Geometry: see drawing. Coordinates: mm, zero at the bounding-box minimum. A direction names the side the tool comes from. Give positions to 0.01 mm unless a question says otherwise; leave off trailing zeros. Write each loop counter-clockwise with the first axis right and the second up, starting at its lowest first coordinate (ties: lowest second). Pieces come first, ordered by that corner, then holes.
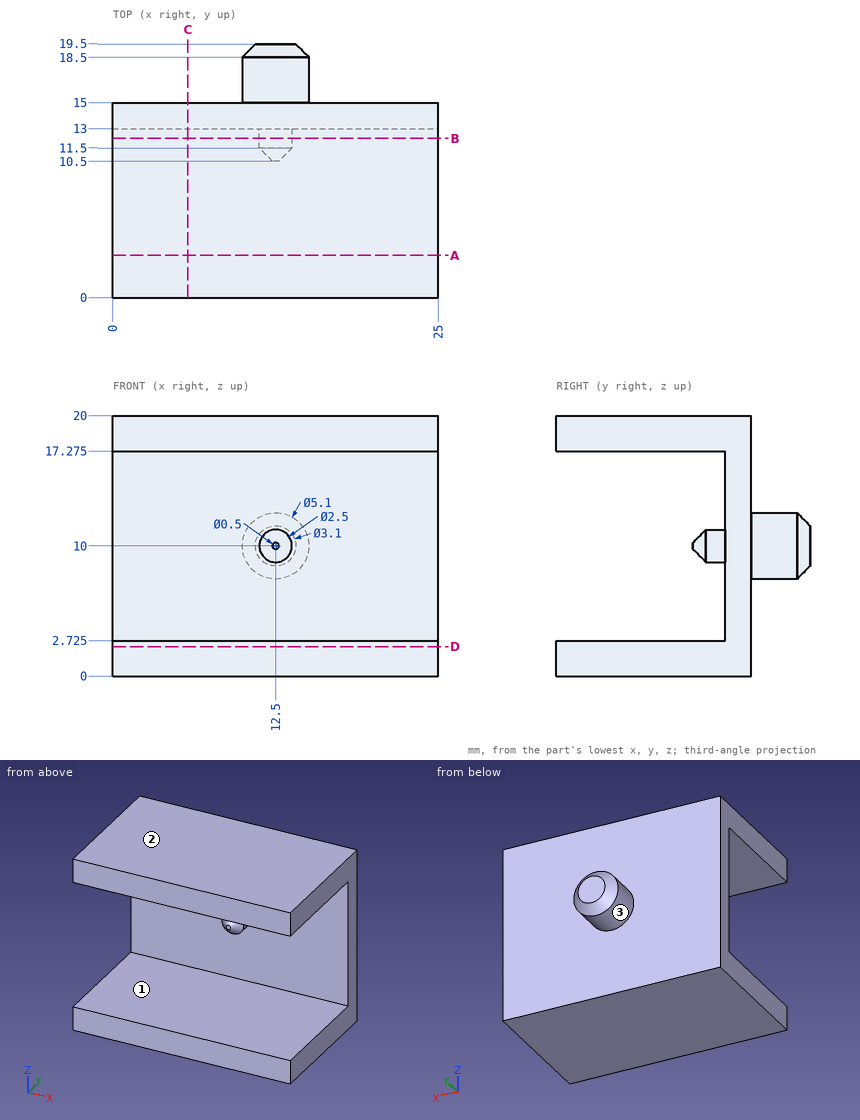
Q1. Section C-C, the plane x = 5.75. Return the cut outline in (y, z) (3 decimals), then the cut area to 3 significant figures.
Q2. Material intervals for line 1 along Z through (x, y) = (19.5, 2.5) (3 decimals); line 2 along Y through (x, z) = (17, 14); line 3 along Y through (x, z) = (8.75, 19.25), sorted ascending.
Q3. Section B-B, the plane y = 12.25. Return the cut outline in (x, z) (3 decimals).
Q4. Access query for the marked faces 1, 2 and 3. Directions: +Z, -Z, +X, -X, +Y, -Y. A direction counts if a zero-diameter tool reaches every point of the face in a straight line with its end or side. Return the directions, or none.
Q5. Pin query (flat end, axial travel): pin 1 (4.5 mm diameter, centred on x = 11, z = 9.5, fed in from -Y); pin 2 (4 mm diameter, centred on x = 8, z = 14.5, fed in from -Y); pin 3 (5 mm diameter, centred on x = 8, z = 16, fed in from +Y). Return the tip coordinate at first contact, or that it passes through.
Q6. Section D-D, the plane z = 2.25. Return the cut outline in (x, y), then the cut area to 3 significant figures.
Q7. Section A-A, the plane y = 3.25. Return the cut outline in (x, z) (3 decimals), then the cut area to 3 significant figures.
Solutions:
1. outline: (0, 0) - (15, 0) - (15, 20) - (0, 20) - (0, 17.275) - (13, 17.275) - (13, 2.725) - (0, 2.725) - close
1. area: 111 mm2
2. line 1: z = 0 to 2.725, 17.275 to 20
2. line 2: y = 13 to 15
2. line 3: y = 0 to 15
3. outline: (0, 0) - (25, 0) - (25, 2.725) - (0, 2.725) - close; (0, 17.275) - (25, 17.275) - (25, 20) - (0, 20) - close; circle Ø2.5 at (12.5, 10)
4. face 1: +X, -X, -Y
4. face 2: +Z, +X, -X, +Y, -Y
4. face 3: +Y
5. pin 1: stops at y = 10.5
5. pin 2: stops at y = 13
5. pin 3: stops at y = 15
6. outline: (0, 0) - (25, 0) - (25, 15) - (0, 15) - close
6. area: 375 mm2
7. outline: (0, 0) - (25, 0) - (25, 2.725) - (0, 2.725) - close; (0, 17.275) - (25, 17.275) - (25, 20) - (0, 20) - close
7. area: 136 mm2
